Work out the finished part from the listing and answer in its coordinate system (mm). A direction names the side the tool comes from. Give positions to 0.01 mm unless a question says otherwise; leave off trailing zeros. Use a Markdown table: item, result. Add a question column.
Q1. For faces 1 (the face through (32, 0, 7)), 2 (the face through (1, -21, -16.5)), 3 (the face through (1, -25, 0)), 4 (the face through (1, -16, 25)), 5 (the face through (-31, 0, -8)), determine the directions among +Z, -Z, +X, -X, +Y, -Y from which every point of the face is accessible in a straight line to the end or side of a thin tool.
Q2. Each of these flat-tipped pins is pushed along its axis until it touches: pin 1 Ø5 at (x, z) = (35, 17.5) entering from +Y; pin 2 Ø1 at (x, y) = (-5.5, -17.5) entering from +Z; pin 3 Ø4 at (y, z) = (14.5, 1) entering from -X. Where does it stop, or does it pass through?
Q3. For a pull along X with two mould halves and no side action, classify faces 6 (the face through (-51.5, -10, 0)), 7 (the face through (31.055, -12.325, -0.846)), 8 (the face through (1, -16, -24)), 9 (the face through (-31.055, -12.325, -0.846)) as pulls with the +X half, pulls with the -X half, needs draft (parallel to the pull), parting line crosses it, or undercut.
Q4. Consider line 1 (X direction, y = -11, z = 0); line 2 (X direction, y = -4.75, z = 0); line 3 (Z direction, x = 37.5, y = -12.25). Determine where each line is inside the solid, lowest interval first.
Q5. Section A-A, the plane z = 0 is taken. State how many separate pieces and enclosed holes the cut face has, plus the area to 3 significant figures.
from build123d import *

# Parameters (mm, degrees)
BOSS_EXTRUDE1_DEPTH = 51.5
SKETCH2_R           = 6.5
CUT_EXTRUDE1_DEPTH  = 66.829324772
BOSS_EXTRUDE4_DEPTH = 75.055534995
SKETCH7_R           = 8
CUT_EXTRUDE3_DEPTH  = 86.666666667


with BuildPart() as part:
    # Sketch1 → Boss-Extrude1 (new, symmetric)
    with BuildSketch(Plane(origin=(0, 0, 0), x_dir=(0, 0, -1), z_dir=(1, 0, 0))):
        Polygon((32.5, 0), (-32.5, 0), (-32.5, -16), (-16.5, -16), (-16.5, -25), (16.5, -25), (16.5, -16), (32.5, -16), align=None)
    extrude(amount=BOSS_EXTRUDE1_DEPTH, both=True)

    # Sketch2 → Cut-Extrude1 (cut, through all)
    with BuildSketch(Plane(origin=(0, 0, 0), x_dir=(1, 0, 0), z_dir=(0, 1, 0))):
        with Locations(Location((-37.5, 0, 0), (0, 0, 270))):
            Circle(SKETCH2_R)
    cut_extrude1 = extrude(amount=-CUT_EXTRUDE1_DEPTH, mode=Mode.SUBTRACT)

    # Mirror1: Cut-Extrude1 across plane
    add(cut_extrude1.mirror(Plane(origin=(0, 0, 0), x_dir=(0, 0, 1), z_dir=(1, 0, 0))), mode=Mode.SUBTRACT)

    # Sketch5 → Boss-Extrude4 (add, along a direction that is not the sketch's normal)
    with BuildSketch(Plane.XY.offset(32.5)):
        with BuildLine():
            Line((0.5, 0), (-37.5, 0))
            ThreePointArc((-37.5, 0), (-18.5, 19), (0.5, 0))
        make_face()
    extrude(amount=-BOSS_EXTRUDE4_DEPTH, dir=(-0.5000000000000041, 0, 0.8660254037844363))

    # Sketch7 → Cut-Extrude3 (cut, along a direction that is not the sketch's normal)
    with BuildSketch(Plane.XY.offset(32.5)):
        with Locations((-18.5, 0)):
            Circle(SKETCH7_R)
    extrude(amount=-CUT_EXTRUDE3_DEPTH, dir=(-0.5000000000000041, 0, 0.8660254037844363), mode=Mode.SUBTRACT)


solid = part.part
Result set:
| question | item | result |
|---|---|---|
| 1 | face 1 | +Z, +X, +Y |
| 1 | face 2 | -Z, +X, -X, -Y |
| 1 | face 3 | +Z, -Z, +X, -X, -Y |
| 1 | face 4 | +Z, +X, -X, -Y |
| 1 | face 5 | -Z, -X, +Y |
| 2 | pin 1 | stops at y = 0 |
| 2 | pin 2 | stops at z = 16.5 |
| 2 | pin 3 | stops at x = -14.96 |
| 3 | face 6 | pulls with the -X half |
| 3 | face 7 | undercut |
| 3 | face 8 | needs draft |
| 3 | face 9 | undercut |
| 4 | line 1 | x = -51.5 to -44, -31 to 31, 44 to 51.5 |
| 4 | line 2 | x = -51.5 to -44, -31 to -6.17, 6.7 to 31, 44 to 51.5 |
| 4 | line 3 | z = -32.5 to -6.5, 6.5 to 32.5 |
| 5 | separate pieces | 3 |
| 5 | enclosed holes | 1 |
| 5 | area | 2,290 mm2 |
